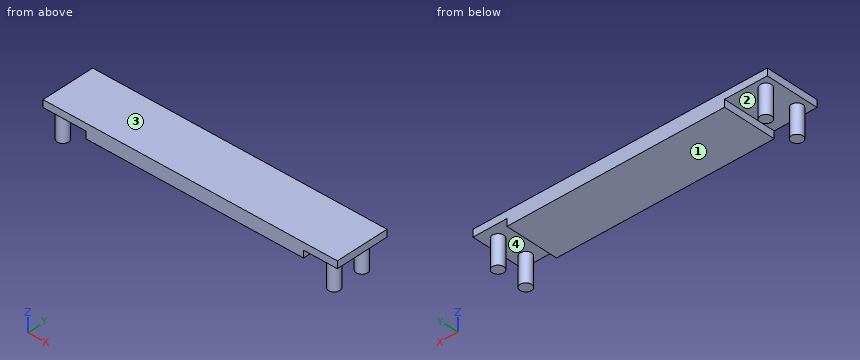
from build123d import *

# Parameters (mm, degrees)
CYLINDER_R        = 1.6
CYLINDER_DEPTH    = 10
BOX001_W          = 61
BOX001_H          = 15
BOX001_DEPTH      = 2
BOX_W             = 82.5
BOX_H             = 15
BOX_DEPTH         = 2
CYLINDER003_R     = 1.6
CYLINDER003_DEPTH = 10
CYLINDER002_R     = 1.6
CYLINDER002_DEPTH = 10
CYLINDER001_R     = 1.6
CYLINDER001_DEPTH = 10


with BuildPart() as taladro1:
    # Cylinder → Cylinder (new body)
    with BuildSketch(Plane(origin=(0, 1.2, -10), x_dir=(1, 0, 0), z_dir=(0, 0, 1))):
        Circle(CYLINDER_R)
    extrude(amount=CYLINDER_DEPTH)


with BuildPart() as perfora_2mm_centro:
    # Box001 → Box001 (new body)
    with BuildSketch(Plane(origin=(12, 0, -2), x_dir=(1, 0, 0), z_dir=(0, 0, 1))):
        with Locations((30.5, 7.5)):
            Rectangle(BOX001_W, BOX001_H)
    extrude(amount=BOX001_DEPTH)


with BuildPart() as fusion001:
    # Box → Box (new body)
    with BuildSketch(Plane.XY):
        with Locations((41.25, 7.5)):
            Rectangle(BOX_W, BOX_H)
    extrude(amount=BOX_DEPTH)

    # Fusion: union perfora_2mm_centro
    add(perfora_2mm_centro.part)


with BuildPart() as fusion001_1:
    # Fusion placement: moved
    add(fusion001.part.moved(Location((-3, -11, -2))))

    # Fusion001: union taladro1
    add(taladro1.part)


with BuildPart() as fusion002:
    # Cylinder003 → Cylinder003 (new body)
    with BuildSketch(Plane(origin=(76, 0.2, -10), x_dir=(1, 0, 0), z_dir=(0, 0, 1))):
        Circle(CYLINDER003_R)
    extrude(amount=CYLINDER003_DEPTH)

    # Fusion002: union Fusion001
    add(fusion001_1.part)


with BuildPart() as fusion003:
    # Cylinder002 → Cylinder002 (new body)
    with BuildSketch(Plane(origin=(76, -8.2, -10), x_dir=(1, 0, 0), z_dir=(0, 0, 1))):
        Circle(CYLINDER002_R)
    extrude(amount=CYLINDER002_DEPTH)

    # Fusion003: union Fusion002
    add(fusion002.part)


with BuildPart() as fusion008:
    # Cylinder001 → Cylinder001 (new body)
    with BuildSketch(Plane(origin=(0, -8.2, -10), x_dir=(1, 0, 0), z_dir=(0, 0, 1))):
        Circle(CYLINDER001_R)
    extrude(amount=CYLINDER001_DEPTH)

    # Fusion008: union Fusion003
    add(fusion003.part)


solid = fusion008.part
Work out the finished part from the listing and answer in its coordinate system (mm). Face numbers are marked on the shaded views. A direction names the side the tool comes from. Give positions to 0.01 mm unless a question says otherwise; leave off trailing zeros. Loops run counter-clockwise (first coordinate to the right, second up) from the corner with the lowest first, then second, coordinate; pieces in that order, holes last. Notation, with made-up numbers: (-14, 83.5) -> (2, 83.5) arc R28 cw to (2, 112.5) -> close; hole circle Ø3 at (81, 16). An arc over 180 degrees is marked (long way). Use a Markdown table: item, result. Add a question column.
1. Flat-ended cylindrical pins translate along their axes: pin 1 Ø6 at (x, y) = (43, -5) entering from -Z; pin 2 Ø1.6 at (y, z) = (-3, -3) entering from +X; pin 3 Ø7.5 at (x, y) = (76, -2) entering from -Z; pin 4 Ø6 at (y, z) = (-9, -6) entering from -X. Find the tip coordinate at first contact, or state that the pin passes through.
2. For the marked faces 1 and 2, determine the directions among +Z, -Z, +X, -X, +Y, -Y from which every point of the face is accessible in a straight line to the end or side of a thin tool.
3. Section D-D on y = -8.2 is taken. Determine the outline of the cut face in (x, z).
4. Section A-A on x = 76 is taken. Determine the outline of the cut face in (y, z).
5. Determine the mould class of the marked faces 3 and 4 for opening direction X: released by +X, released by -X, zero draft, split by the parting line, or undercut.
6. Find the intervals of material crossed by probe 1 along Z at (x, y) = (51, 2.75); probe 2 along Z at (x, y) = (74, -4); probe 3 along X at (y, z) = (0, -7.5), in increasing order.
7. Section B-B on y = -3 is taken. Determine the outline of the cut face in (x, z).
8. Section C-C on z = -8.75 is taken. Determine the outline of the cut face in (x, y).
Results below:
| question | item | result |
|---|---|---|
| 1 | pin 1 | stops at z = -4 |
| 1 | pin 2 | stops at x = 70 |
| 1 | pin 3 | stops at z = -10 |
| 1 | pin 4 | stops at x = -1.6 |
| 2 | face 1 | -Z, +Y, -Y |
| 2 | face 2 | -Z |
| 3 | outline | (-3, -2) -> (-1.6, -2) -> (-1.6, -10) -> (1.6, -10) -> (1.6, -2) -> (9, -2) -> (9, -4) -> (70, -4) -> (70, -2) -> (74.4, -2) -> (74.4, -10) -> (77.6, -10) -> (77.6, -2) -> (79.5, -2) -> (79.5, 0) -> (-3, 0) -> close |
| 4 | outline | (-11, -2) -> (-9.8, -2) -> (-9.8, -10) -> (-6.6, -10) -> (-6.6, -2) -> (-1.4, -2) -> (-1.4, -10) -> (1.8, -10) -> (1.8, -2) -> (4, -2) -> (4, 0) -> (-11, 0) -> close |
| 5 | face 3 | zero draft |
| 5 | face 4 | undercut |
| 6 | probe 1 | z = -4 to 0 |
| 6 | probe 2 | z = -2 to 0 |
| 6 | probe 3 | x = -1.06 to 1.06, 74.41 to 77.59 |
| 7 | outline | (-3, -2) -> (9, -2) -> (9, -4) -> (70, -4) -> (70, -2) -> (79.5, -2) -> (79.5, 0) -> (-3, 0) -> close |
| 8 | outline | circle Ø3.2 at (0, -8.2); circle Ø3.2 at (0, 1.2); circle Ø3.2 at (76, -8.2); circle Ø3.2 at (76, 0.2) |
